Verification items for this drawing (mm, ordinates from the low corner). A direction names the side the tool comes from. Coordinates: 2 decimals unless noted, no trailing zeros. Order: outer loops, then holes, each group sorted by start corner. A loop starts at its lowest first (then second) coordinate and runs counter-clockwise, first axis right, second up. Notation, with made-up numbers: (63.5, 67) -> (111.5, 67) arc R20 cw to (111.5, 75) -> close; hole circle Ø7 at (-27, 5.25). An arc over 180 degrees is marked (long way). Write each question's results on one line, items separated by ' | '. Start each with the question number.
(1) Cross-section at B-B on y = 4. Enter the section's corners in (x, z), and give its area (3 significant figures).
(2) Thickness scan on probe 1 along Y at (x, z) = (5, 15); probe 2 along Z at (x, y) = (18, 1.25) (1 decimal); probe 3 along Y at (x, z) = (20, 19.5). Record the ranges inside material, lowest first. Write a range as [from, to].
(3) Cross-section at A-A on z = 12.6. Enter the section's corners in (x, y), and give its area (3 significant figures).
(4) Set-up check for the marked faces 1, 2 and 3: record each of +Z, -Z, +X, -X, +Y, -Y from which the full face is reachable in a straight line by a thin tool's end or side.
(5) Cross-section at D-D on y = 14.25. Enter the section's corners in (x, z).
(6) Go/stop test with flat-tipped pins: pin 1 (5 mm diameter, centred on x = 16.5, y = 7.5, fed in from +Z); pin 2 (5 mm diameter, centred on y = 10, z = 5.5, fed in from -X); pin 3 (2 mm diameter, centred on y = 5.5, z = 20.5, fed in from -X). Record where each tip stops, or that it passes through.
(7) Cross-section at C-C on x = 12. Enter the section's corners in (y, z), and give its area (3 significant figures).
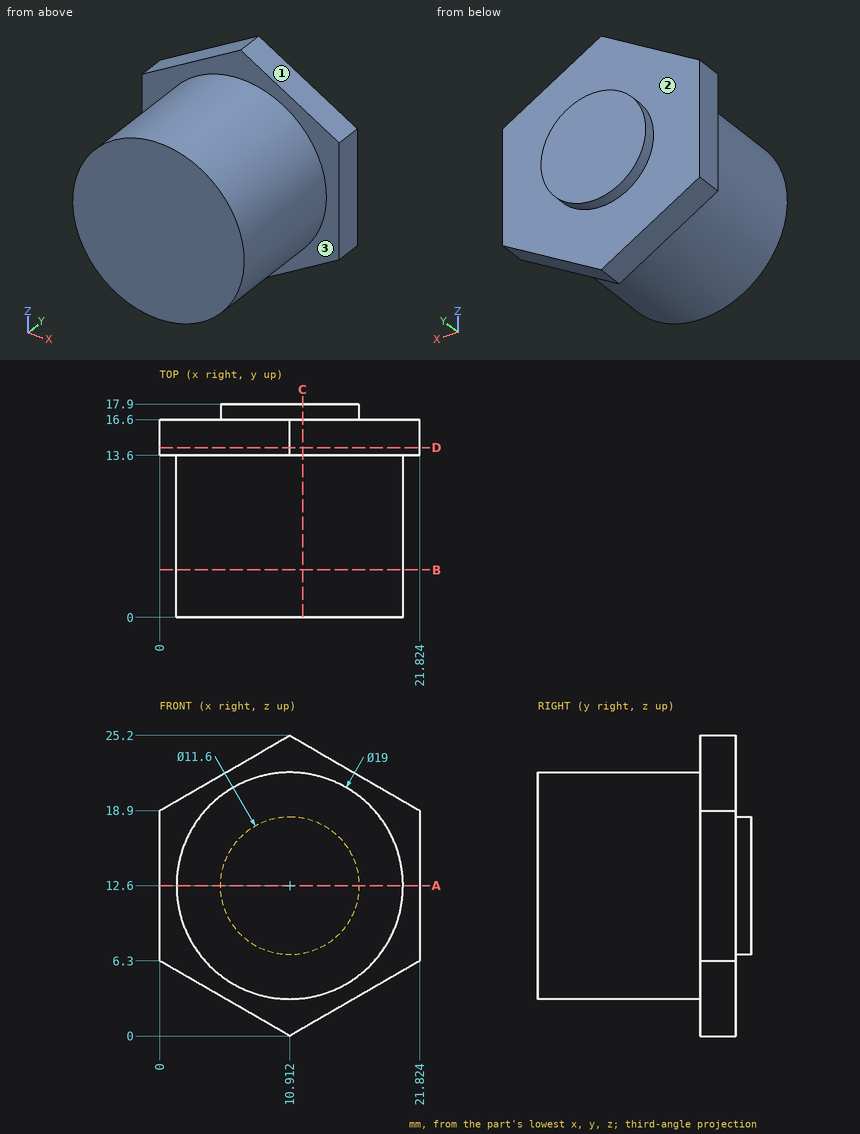
Results are:
1) outline: circle Ø19 at (10.91, 12.6) | area: 284 mm2
2) probe 1: y = [0, 16.6] | probe 2: z = [6.3, 18.9] | probe 3: y = [13.6, 16.6]
3) outline: (0, 13.6) -> (1.41, 13.6) -> (1.41, 0) -> (20.41, 0) -> (20.41, 13.6) -> (21.82, 13.6) -> (21.82, 16.6) -> (16.71, 16.6) -> (16.71, 17.9) -> (5.11, 17.9) -> (5.11, 16.6) -> (0, 16.6) -> close | area: 339 mm2
4) face 1: +Z, +X, +Y, -Y | face 2: +Y | face 3: -Y
5) outline: (0, 6.3) -> (10.91, 0) -> (21.82, 6.3) -> (21.82, 18.9) -> (10.91, 25.2) -> (0, 18.9) -> close
6) pin 1: stops at z = 21.58 | pin 2: stops at x = 2.6 | pin 3: stops at x = 4.38
7) outline: (0, 3.16) -> (13.6, 3.16) -> (13.6, 0.63) -> (16.6, 0.63) -> (16.6, 6.9) -> (17.9, 6.9) -> (17.9, 18.3) -> (16.6, 18.3) -> (16.6, 24.57) -> (13.6, 24.57) -> (13.6, 22.04) -> (0, 22.04) -> close | area: 343 mm2
